from build123d import *

# Parameters (mm, degrees)
SKETCH1_W           = 70
SKETCH1_H           = 70
BOSS_EXTRUDE1_DEPTH = 47
FILLET1_R           = 20
SHELL1_T            = -2
SKETCH2_R           = 21.5
CUT_EXTRUDE1_DEPTH  = 69.256867786
SKETCH6_W           = 75
SKETCH6_H           = 43.024157236
CUT_EXTRUDE4_DEPTH  = 69.256867786
SKETCH7_W           = 25.54869255
SKETCH7_H           = 28.800793666
CUT_EXTRUDE5_DEPTH  = 10
SKETCH9_W           = 25.672093796
SKETCH9_H           = 28.560455229
CUT_EXTRUDE6_DEPTH  = 10


with BuildPart() as part:
    # Sketch1 → Boss-Extrude1 (new body)
    with BuildSketch(Plane(origin=(0, 0, 0), x_dir=(1, 0, 0), z_dir=(0, 1, 0))):
        Rectangle(SKETCH1_W, SKETCH1_H)
    extrude(amount=BOSS_EXTRUDE1_DEPTH)

    # Fillet1
    fillet1_edges = [part.edges().sort_by_distance(p)[0] for p in [
        (35, 23.5, 35),
        (-35, 23.5, 35),
        (-35, 23.5, -35),
        (35, 23.5, -35),
    ]]
    fillet(fillet1_edges, radius=FILLET1_R)

    # Shell1
    shell1_openings = [part.faces().sort_by_distance(p)[0] for p in [
        (0, 0, 0),
    ]]
    offset(amount=SHELL1_T, openings=shell1_openings, kind=Kind.INTERSECTION)

    # Sketch2 → Cut-Extrude1 (cut, through all)
    with BuildSketch(Plane(origin=(0, 47, 0), x_dir=(1, 0, 0), z_dir=(0, 1, 0))):
        with Locations(Location((5, -5, 0), (0, 0, 270))):
            Circle(SKETCH2_R)
    extrude(amount=-CUT_EXTRUDE1_DEPTH, mode=Mode.SUBTRACT)

    # Sketch6 → Cut-Extrude4 (cut, through all)
    with BuildSketch(Plane(origin=(0, 0, 0), x_dir=(0.7071067811865477, 0, -0.7071067811865475), z_dir=(0.7071067811865475, 0, 0.7071067811865477))):
        with Locations((0, 21.512078618)):
            Rectangle(SKETCH6_W, SKETCH6_H)
    extrude(amount=CUT_EXTRUDE4_DEPTH, mode=Mode.SUBTRACT)

    # Sketch7 → Cut-Extrude5 (cut)
    with BuildSketch(Plane(origin=(0, 0, -35), x_dir=(-1, 0, 0), z_dir=(0, 0, -1))):
        with Locations((-5.439128437, 14.400396833)):
            Rectangle(SKETCH7_W, SKETCH7_H)
    extrude(amount=-CUT_EXTRUDE5_DEPTH, mode=Mode.SUBTRACT)

    # Sketch9 → Cut-Extrude6 (cut)
    with BuildSketch(Plane.ZY.offset(35)):
        with Locations((5.425785495, 14.280227615)):
            Rectangle(SKETCH9_W, SKETCH9_H)
    extrude(amount=-CUT_EXTRUDE6_DEPTH, mode=Mode.SUBTRACT)


solid = part.part
Verification items for the finished model (mm, model axes). A direction names the side the tool comes from. Give positions to 0.01 mm unless a question says otherwise; leave off trailing zeros. Loops run counter-clockwise (first coordinate to the right, second up) from the corner with the lowest first, then second, coordinate; pieces in that order, holes last.
1. Cross-section at B-B on x = 5. Record the cut outline in (y, z), and give its area (4 significant figures).
Derived:
outline: (28.8, -35) - (47, -35) - (47, -16.5) - (45, -16.5) - (45, -33) - (28.8, -33) - close; (43.02, 33) - (45, 33) - (45, 26.5) - (47, 26.5) - (47, 35) - (43.02, 35) - close
area: 90.35 mm2
2. Cross-section at C-C on z = -11. Record the cut outline in (x, y).
Derived:
outline: (-35, 0) - (-33, 0) - (-33, 45) - (-9.36, 45) - (-9.36, 47) - (-35, 47) - close; (19.36, 45) - (33, 45) - (33, 43.02) - (35, 43.02) - (35, 47) - (19.36, 47) - close
3. Go/stop test with flat-tipped pins: P1, Ø10, axis at y = 6.5, z = -20, coming from the +X side; P2, Ø1.1, axis at x = -34, z = 1.5, coming from the -Y side; P3, Ø4, axis at x = -19, y = 6.5, coming from the -Z side; P4, Ø12, axis at x = 23.5, z = 2, coming from the +Y side. Record where each tip stops, or that it passes through.
Derived:
P1: stops at x = 34.72
P2: stops at y = 28.56
P3: stops at z = -34.9
P4: stops at y = 47
4. Cross-section at A-A on y = 13. Record the cut outline in (x, z).
Derived:
outline: (-35, -15) arc R20 ccw to (-15, -35) - (-7.34, -35) - (-7.34, -33) - (-15, -33) arc R18 cw to (-33, -15) - (-33, -7.41) - (-35, -7.41) - close; (-34.73, 18.26) - (-32.7, 18.26) arc R18 cw to (-21.1, 31.94) - (-18.31, 34.72) arc R20 ccw to start; (18.21, -34.74) arc R20 ccw to (34.72, -18.31) - (31.94, -21.1) arc R18 cw to (18.21, -32.71) - close
5. Cross-section at D-D on y = 41. Record the cut outline in (x, z), and give its area (3 significant figures).
Derived:
outline: (-35, -15) arc R20 ccw to (-15, -35) - (15, -35) arc R20 ccw to (34.72, -18.31) - (31.94, -21.1) arc R18 cw to (15, -33) - (-15, -33) arc R18 cw to (-33, -15) - (-33, 15) arc R18 cw to (-21.1, 31.94) - (-18.31, 34.72) arc R20 ccw to (-35, 15) - close
area: 280 mm2
6. Tool access check on faces 1 (the flat face through (-19.722, 21.211, 33.311)), 2 (the flat face through (-34, 14, -7.41)), 3 (the flat face through (6, 28.801, -34)). Record the directions out of +Z, -Z, +X, -X, +Y, -Y that give a thin tool (end or side, any length) a straight path to the whole face; none if there is none.
Derived:
face 1: +X, -Y
face 2: +X, -X, -Y
face 3: +Z, -Z, -Y
7. Material ranges on probe 1 along X at (y, z) = (46, 5); probe 2 along Z at (x, y) = (-15, 14); probe 3 along Y at (x, z) = (-25.5, 12.5), recorded low to high.
Derived:
probe 1: x = -35 to -16.5, 26.5 to 35
probe 2: z = -35 to -33
probe 3: y = 45 to 47
8. Release check for a two-part mould opening along Z. For faces 4 (the flat face through (33.311, 21.211, -19.722)), 5 (the flat face through (-34, 14, 18.262)), 6 (the flat face through (-0.5, 47, -16)) record: +Z half, -Z half, draft (parallel to the pull), parting line (faces both ways), or undercut.
Derived:
face 4: +Z half
face 5: undercut
face 6: draft
